```python
from build123d import *

# Parameters (mm, degrees)
EXTRUDE_START      = 300
EXTRUDE_SKETCH_1_R = 82
EXTRUDE_1_DEPTH    = 3


with BuildPart() as part:
    # Extrude sketch 1 → Extrude 1 (new body)
    with BuildSketch(Plane.XY.offset(EXTRUDE_START)):
        with BuildLine():
            Line((871, 170), (114, 170))
            ThreePointArc((114, 170), (104.100505063, 165.899494937), (100, 156))
            Line((100, 156), (100, -156))
            ThreePointArc((100, -156), (104.100505063, -165.899494937), (114, -170))
            Line((114, -170), (871, -170))
            ThreePointArc((871, -170), (880.899494937, -165.899494937), (885, -156))
            Line((885, -156), (885, 156))
            ThreePointArc((885, 156), (880.899494937, 165.899494937), (871, 170))
        make_face()
        with Locations((240, 0)):
            Circle(EXTRUDE_SKETCH_1_R, mode=Mode.SUBTRACT)
    extrude(amount=EXTRUDE_1_DEPTH)


solid = part.part
```
Could you check a few things on this model? Use its own coordinates, in mm. Coordinates: 2 decimals unless noted, no trailing zeros. Order: outer loops, then holes, each group sorted by start corner. A loop starts at its lowest first (then second) coordinate and runs counter-clockwise, first axis right, second up. Notation, with made-up numbers: M 34,61 L 42,61 A32 cw 42,98 Z; hole C 63,-13 d9. An arc over 180 degrees is marked long. Use a Markdown table: item, result. Add a question column.
Q1. I want a section at B-B on y = 0. List the corners of the cut face in (x, z) for me, then the cut area to 3 significant figures.
Q2. We'd pull the mould along X, two halves only. Please class faces 1 (the flat face through (487, 2, 300)), 2 (the cylindrical face through (104, -165.8, 301.5)), 3 (the cylindrical face through (880.8, -166, 301.5)), 4 (the cylindrical face through (318.213, 24.631, 301.479)): pulls with the +X half, pulls with the -X half, needs draft (parallel to the pull), parting line crosses it, or undercut.
Q3. I want a section at C-C on z = 301.95. List the corners of the cut face in (x, y) for me, then the cut area to 3 significant figures.
Q4. If I drill on L1, parallel to Y at x = 240, z = 300.9; L2, parallel to X at y = 61, z = 302.8; L3, parallel to X at y = 7, z = 300.75, over which ranges is the centre line in solid material (lowest first)?
Q5. I want a section at A-A on x = 240. List the corners of the cut face in (y, z) for me, then the cut area to 3 significant figures.
Checked values:
| question | item | result |
|---|---|---|
| 1 | outline | M 100,300 L 158,300 L 158,303 L 100,303 Z; M 322,300 L 885,300 L 885,303 L 322,303 Z |
| 1 | area | 1,860 mm² |
| 2 | face 1 | needs draft |
| 2 | face 2 | pulls with the -X half |
| 2 | face 3 | pulls with the +X half |
| 2 | face 4 | undercut |
| 3 | outline | M 100,-156 A14 ccw 114,-170 L 871,-170 A14 ccw 885,-156 L 885,156 A14 ccw 871,170 L 114,170 A14 ccw 100,156 Z; hole C 240,0 d164 |
| 3 | area | 246,000 mm² |
| 4 | L1 | -170 to -82, 82 to 170 |
| 4 | L2 | 100 to 185.2, 294.8 to 885 |
| 4 | L3 | 100 to 158.3, 321.7 to 885 |
| 5 | outline | M -170,300 L -82,300 L -82,303 L -170,303 Z; M 82,300 L 170,300 L 170,303 L 82,303 Z |
| 5 | area | 528 mm² |
